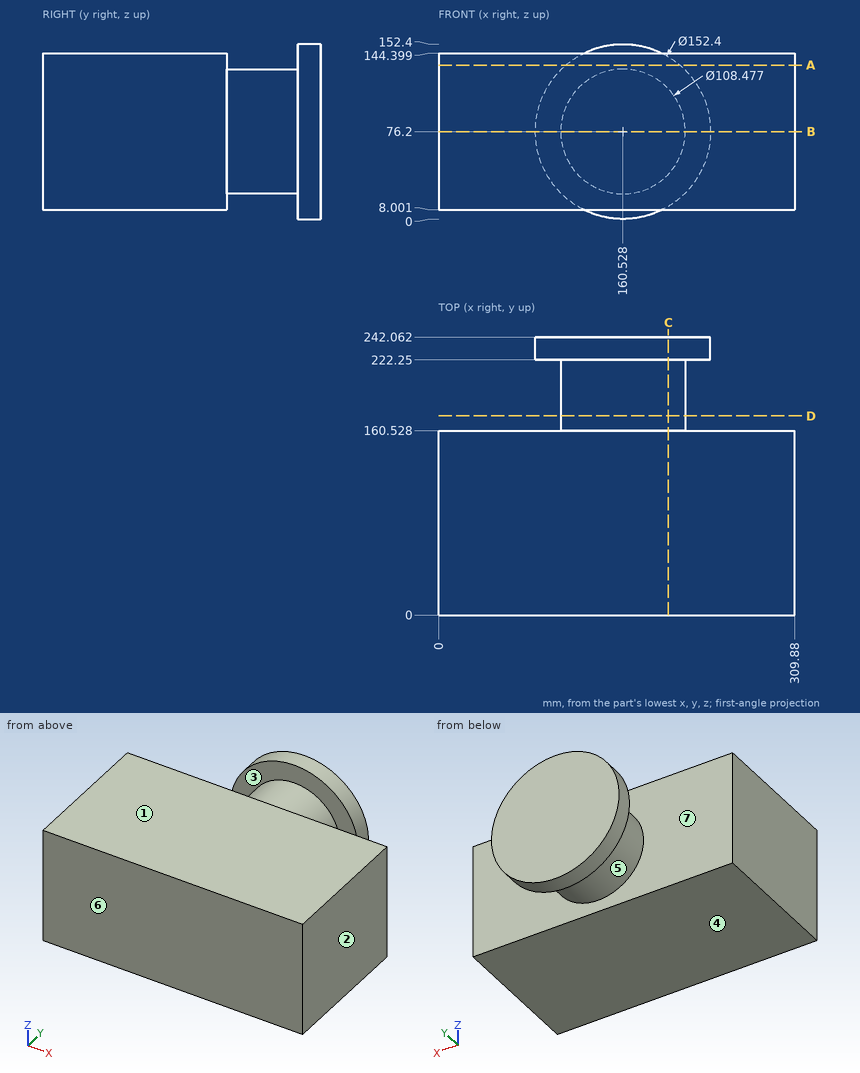
Answer from the drawing. Dimensions are ordinates in mm from the lowest x, y and z of the part. A direction names the side the tool comes from. Round coordinates to 2 decimals unless told otherwise and drop trailing zeros. Loops run counter-clockwise (first coordinate to the right, second up) from the corner with the lowest first, then second, coordinate; pieces in that order, holes last.
(1) Each of these flat-tipped pins is pushed along its axis until it touches: P1, Ø5, axis at y = 204.5, z = 32.5, coming from the -X side; P2, Ø12, axis at y = 202, z = 93.5, coming from the -X side; P3, Ø12, axis at x = 67.5, y = 82, coming from the -Z side. Where does it stop, or does it pass through?
Computed values:
P1: stops at x = 125.25
P2: stops at x = 107.48
P3: stops at z = 8
(2) Find the intervals of material crossed by L1, parallel to Y at x = 212, z = 99; L2, parallel to Z at x = 20, y = 135.5; L3, parallel to Y at x = 104.5, z = 23, in increasing order.
Computed values:
L1: y = 0 to 160.53, 222.25 to 242.06
L2: z = 8 to 144.4
L3: y = 0 to 160.53
(3) The part is cut by section B-B, the plane z = 76.2. Give the vertices of the cut face in (x, y).
Computed values:
outline: (0, 0) - (309.88, 0) - (309.88, 160.53) - (214.77, 160.53) - (214.77, 222.25) - (236.73, 222.25) - (236.73, 242.06) - (84.33, 242.06) - (84.33, 222.25) - (106.29, 222.25) - (106.29, 160.53) - (0, 160.53) - close
(4) The part is cut by section C-C, the plane x = 200. Give the vertices of the cut face in (y, z).
Computed values:
outline: (0, 8) - (160.53, 8) - (160.53, 39) - (222.25, 39) - (222.25, 11.02) - (242.06, 11.02) - (242.06, 141.38) - (222.25, 141.38) - (222.25, 113.4) - (160.53, 113.4) - (160.53, 144.4) - (0, 144.4) - close
(5) The part is cut by section A-A, the plane z = 134. Give the vertices of the cut face in (x, y), and give its area (3 significant figures).
Computed values:
outline: (0, 0) - (309.88, 0) - (309.88, 160.53) - (0, 160.53) - close; (110.87, 222.25) - (210.18, 222.25) - (210.18, 242.06) - (110.87, 242.06) - close
area: 51,700 mm2
(6) The mould has two halves that part along Y. Classify the marked faces 4, 5, 6 and 7: pulls with the +Y half, pulls with the -Y half, needs draft (parallel to the pull), parting line crosses it, or undercut.
Computed values:
face 4: needs draft
face 5: undercut
face 6: pulls with the -Y half
face 7: undercut
(7) For the marked faces 1, 2 and 3, determine the directions among +Z, -Z, +X, -X, +Y, -Y from which every point of the face is accessible in a straight line to the end or side of a thin tool.
Computed values:
face 1: +Z, +X, -X, -Y
face 2: +Z, -Z, +X, +Y, -Y
face 3: none
(8) The part is cut by section D-D, the plane y = 173.5. Give the vertices of the cut face in (x, z).
Computed values:
outline: circle Ø108.48 at (160.53, 76.2)
